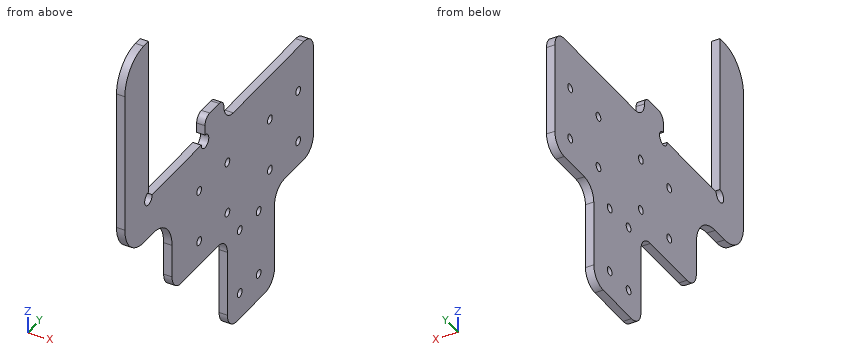
from build123d import *

# Parameters (mm, degrees)
F0_R     = 2.5
F1_DEPTH = 5


with BuildPart() as f1:
    # F0 (on Right) → F1 (new body)
    with BuildSketch(Plane.YZ):
        with BuildLine():
            Line((43.73, -37.5), (65, -37.5))
            ThreePointArc((65, -37.5), (72.071068, -34.571068), (75, -27.5))
            Line((75, -27.5), (75, 27.5))
            ThreePointArc((75, 27.5), (72.071068, 34.571068), (65, 37.5))
            Line((65, 37.5), (-10, 37.5))
            ThreePointArc((-10, 37.5), (-17.071068, 40.428932), (-20, 47.5))
            ThreePointArc((-20, 47.5), (-21.464466, 51.035534), (-25, 52.5))
            Line((-25, 52.5), (-35, 52.5))
            ThreePointArc((-35, 52.5), (-38.535534, 51.035534), (-40, 47.5))
            Line((-40, 47.5), (-40, 41.5))
            ThreePointArc((-40, 41.5), (-37.171573, 34.671573), (-44, 37.5))
            Line((-44, 37.5), (-96, 37.5))
            ThreePointArc((-96, 37.5), (-102.828427, 34.671573), (-100, 41.5))
            Line((-100, 41.5), (-100, 137.5))
            Line((-100, 137.5), (-105, 137.5))
            ThreePointArc((-105, 137.5), (-119.142136, 131.642136), (-125, 117.5))
            Line((-125, 117.5), (-125, 32.5))
            ThreePointArc((-125, 32.5), (-119.142136, 18.357864), (-105, 12.5))
            Line((-105, 12.5), (-95, 12.5))
            ThreePointArc((-95, 12.5), (-80.857864, 6.642136), (-75, -7.5))
            Line((-75, -7.5), (-75, -27.5))
            ThreePointArc((-75, -27.5), (-72.071068, -34.571068), (-65, -37.5))
            Line((-65, -37.5), (-26.27, -37.5))
            ThreePointArc((-26.27, -37.5), (-19.198932, -40.428932), (-16.27, -47.5))
            Line((-16.27, -47.5), (-16.27, -87.5))
            ThreePointArc((-16.27, -87.5), (-13.341068, -94.571068), (-6.27, -97.5))
            Line((-6.27, -97.5), (23.73, -97.5))
            ThreePointArc((23.73, -97.5), (30.801068, -94.571068), (33.73, -87.5))
            Line((33.73, -87.5), (33.73, -47.5))
            ThreePointArc((33.73, -47.5), (36.658932, -40.428932), (43.73, -37.5))
        make_face()
        with Locations((-46.23, -22.27)):
            Circle(F0_R, mode=Mode.SUBTRACT)
        with Locations((-46.23, 9.73)):
            Circle(F0_R, mode=Mode.SUBTRACT)
        with Locations((-3.15, -81.31)):
            Circle(F0_R, mode=Mode.SUBTRACT)
        with Locations((16.85, -81.31)):
            Circle(F0_R, mode=Mode.SUBTRACT)
        with Locations((-3.15, -41.31)):
            Circle(F0_R, mode=Mode.SUBTRACT)
        with Locations((16.85, -41.31)):
            Circle(F0_R, mode=Mode.SUBTRACT)
        with Locations((-16.23, -22.27)):
            Circle(F0_R, mode=Mode.SUBTRACT)
        with Locations((-16.23, 9.73)):
            Circle(F0_R, mode=Mode.SUBTRACT)
        with Locations((28.77, -22.27)):
            Circle(F0_R, mode=Mode.SUBTRACT)
        with Locations((58.77, -22.27)):
            Circle(F0_R, mode=Mode.SUBTRACT)
        with Locations((28.77, 9.73)):
            Circle(F0_R, mode=Mode.SUBTRACT)
        with Locations((58.77, 9.73)):
            Circle(F0_R, mode=Mode.SUBTRACT)
    extrude(amount=F1_DEPTH)


solid = f1.part
Verification items for the finished model (mm, model axes). Give positions to 0.01 mm unless a question says otherwise; leave off trailing zeros. Loops run counter-clockwise (first coordinate to the right, second up) from the corner with the lowest first, then second, coordinate; pieces in that order, holes last.
1. Cross-section at B-B on z = 9.73. Record the cut outline in (x, y), and give its area (3 significant figures).
Derived:
outline: (0, -84.84) - (5, -84.84) - (5, -48.73) - (0, -48.73) - close; (0, -43.73) - (5, -43.73) - (5, -18.73) - (0, -18.73) - close; (0, -13.73) - (5, -13.73) - (5, 26.27) - (0, 26.27) - close; (0, 31.27) - (5, 31.27) - (5, 56.27) - (0, 56.27) - close; (0, 61.27) - (5, 61.27) - (5, 75) - (0, 75) - close
area: 699 mm2
2. Go/stop test with flat-tipped pins: P1, Ø4.5, axis at y = -46.23, z = 9.73, coming from the +X side; P2, Ø3, axis at x = 2.5, y = -35, coming from the -Z side; P3, Ø2.5, axis at x = 2.5, y = -101.5, coming from the -Z side; P4, Ø1.5, axis at x = 1.5, y = 51.5, coming from the +Z side. Record where each tip stops, or that it passes through.
Derived:
P1: passes through
P2: stops at z = -37.5
P3: stops at z = 12.5
P4: stops at z = 37.5
3. Material ranges on probe 1 along Z at (x, y) = (3.45, -3.15); probe 2 along Y at (x, z) = (3.05, -81); probe 3 along Z at (x, y) = (3.2, -46.23), recorded low to high.
Derived:
probe 1: z = -97.5 to -83.81, -78.81 to -43.81, -38.81 to 37.5
probe 2: y = -16.27 to -5.63, -0.67 to 14.37, 19.33 to 33.73
probe 3: z = -37.5 to -24.77, -19.77 to 7.23, 12.23 to 37.5
4. Cross-section at A-A on y = 16.85. Record the cut outline in (x, z), and give its area (3 significant figures).
Derived:
outline: (0, -97.5) - (5, -97.5) - (5, -83.81) - (0, -83.81) - close; (0, -78.81) - (5, -78.81) - (5, -43.81) - (0, -43.81) - close; (0, -38.81) - (5, -38.81) - (5, 37.5) - (0, 37.5) - close
area: 625 mm2
5. Cross-section at D-D on x = 3.6. Count the separate pieces of the cut face and the enclosed holes in it, and give its area (3 significant figures).
Derived:
separate pieces: 1
enclosed holes: 12
area: 17,800 mm2
6. Cross-section at C-C on z = -41.31. Record the cut outline in (x, y).
Derived:
outline: (0, -18.42) - (5, -18.42) - (5, -5.65) - (0, -5.65) - close; (0, -0.65) - (5, -0.65) - (5, 14.35) - (0, 14.35) - close; (0, 19.35) - (5, 19.35) - (5, 35.88) - (0, 35.88) - close
